Could you check a few things on this model? Use its own coordinates, in mm. Face numbers are marked on the shaded views. A direction names the side the tool comes from. Coordinates: 2 decimals unless noted, no trailing zeros. Loops run counter-clockwise (first coordinate to the right, second up) from the corner with the lowest first, then second, coordinate; pieces in that order, holes last.
1) Imagine slicing it at A-A on y = 6.5. Please give me the cut outline in (x, z).
2) Thinking about a two-plate mould opening in Z: for the marked faces 3, 4 and 5, which applies, released by +Z, released by -Z, zero draft, split by the parting line, or undercut?
3) Will these pins go through, and if not, where does the flat tip stop? P1, Ø3, axis at x = -24, y = 10.5, coming from the +Z side; P2, Ø12, axis at x = -13.5, z = -9.5, coming from the +Y side.
4) Imagine slicing it at B-B on x = -20.5. Please give me the cut outline in (y, z).
5) Imagine slicing it at C-C on z = -7. Please give me the cut outline in (x, y).
6) For the marked faces 1 and 2, which set-ups out of +Z, -Z, +X, -X, +Y, -Y let a thin tool reach every point of the face, with its end or its side?
7) If I drill on line 1 along Z through (x, y) = (-28, 8.5); line 2 along Y through (x, z) = (-5, -15.75), over which ranges is the centre line in solid material (lowest first)?
Autodesk Inventor part; units mm, degrees
ref_plane "YZ Plane" through (0, 0, 0) normal (1, 0, 0) x (0, 1, 0)
ref_plane "XZ Plane" through (0, 0, 0) normal (0, 1, 0) x (-1, 0, 0)
ref_plane "XY Plane" through (0, 0, 0) normal (0, 0, 1) x (1, 0, 0)
sketch "Sketch1" plane through (0, 0, 0) normal (0, 1, 0) x (-1, 0, 0)
  line L0 (0, 0) -> (40, 0)
  line L1 (40, 0) -> (40, -28.5)
  line L2 (40, -28.5) -> (0, -28.5)
  line L3 (0, -28.5) -> (0, 0)
  dimension "d0" = 40
  dimension "d1" = 28.5
extrude "Plate1" add sketch "Sketch1" along normal blind 1.5
sketch "Sketch2" plane through (0, 0, -1.5) normal (0, 0, 1) x (1, 0, 0)
  line L0 (-40, 0) -> (0, 0)
  line L1 (0, 0) -> (0, 15)
  line L2 (0, 15) -> (-40, 15)
  line L3 (-40, 15) -> (-40, 0)
edge flange "Flange1" height 15 angle 90 thickness 1.5 bend radius 0.31 thickness toward (0, 0, 1) relief tear relief width 1.5 relief depth 0.75 edges at (-20, 1.5, 0) wall of the first edge with corners at (-40, 0, -1.5) (0, 0, -1.5) (0, 15, -1.5) (-40, 15, -1.5)
bend "Bend1"
corner "Corner1"
sketch "Sketch3" plane through (-40, 0, -27) normal (0, 0, -1) x (-1, 0, 0)
  line L0 (-40, 0) -> (0, 0)
  line L1 (0, 0) -> (0, 15)
  line L2 (0, 15) -> (-40, 15)
  line L3 (-40, 15) -> (-40, 0)
edge flange "Flange2" height 15 angle 90 thickness 1.5 bend radius 0.31 thickness toward (0, 0, -1) relief tear relief width 1.5 relief depth 0.75 edges at (-20, 1.5, -28.5) wall of the first edge with corners at (0, 0, -27) (-40, 0, -27) (-40, 15, -27) (0, 15, -27)
bend "Bend2"
corner "Corner2"
equation "\"d2\" = Thickness"
equation "\"d3\" = BendReliefWidth"
equation "\"d4\" = BendReliefDepth"
equation "\"d5\" = MinimumRemnant"
equation "\"d6\" = TransitionRadius"
equation "\"d9\" = BendRadius"
equation "\"d10\" = CornerReliefSize"
equation "\"d11\" = GapSize"
equation "\"d12\" = JacobiRadiusSize"
equation "\"d13\" = BendReliefWidth"
equation "\"d14\" = BendReliefDepth"
equation "\"d15\" = MinimumRemnant"
equation "\"d16\" = TransitionRadius"
equation "\"d19\" = BendRadius"
equation "\"d20\" = CornerReliefSize"
equation "\"d21\" = GapSize"
equation "\"d22\" = JacobiRadiusSize"
equation "\"BendReliefWidth\" = Thickness"
equation "\"BendReliefDepth\" = 0.5 * Thickness"
equation "\"CornerReliefSize\" = 4 * Thickness"
equation "\"MinimumRemnant\" = 2 * Thickness"
equation "\"TransitionRadius\" = BendRadius"
equation "\"JacobiRadiusSize\" = BendRadius"
equation "\"GapSize\" = Thickness"
properties part number "body_motor_frame" material "Aluminum 6061-AHC"
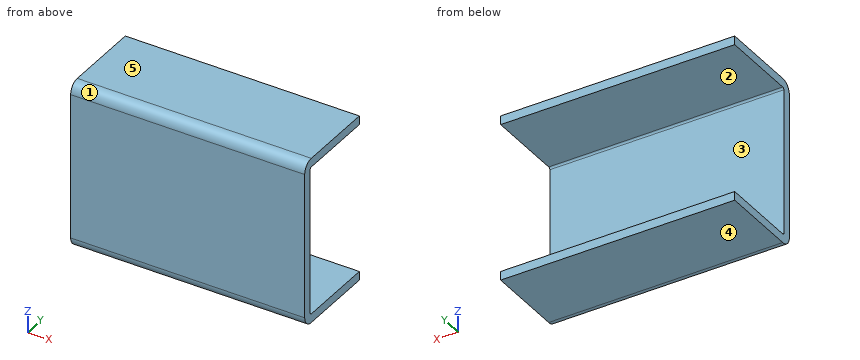
Filled in:
1. outline: (-40, -28.5) - (0, -28.5) - (0, -27) - (-40, -27) - close; (-40, -1.5) - (0, -1.5) - (0, 0) - (-40, 0) - close
2. face 3: undercut
2. face 4: released by -Z
2. face 5: released by +Z
3. P1: stops at z = 0
3. P2: stops at y = 1.5
4. outline: (0, -26.69) arc R1.81 ccw to (1.81, -28.5) - (15, -28.5) - (15, -27) - (1.81, -27) arc R0.31 cw to (1.5, -26.69) - (1.5, -1.81) arc R0.31 cw to (1.81, -1.5) - (15, -1.5) - (15, 0) - (1.81, 0) arc R1.81 ccw to (0, -1.81) - close
5. outline: (-40, 0) - (0, 0) - (0, 1.5) - (-40, 1.5) - close
6. face 1: +Z, +X, -X, -Y
6. face 2: +X, -X, +Y
7. line 1: z = -28.5 to -27, -1.5 to 0
7. line 2: y = 0 to 1.5
